from build123d import *

# Parameters (mm, degrees)
BOSS_EXTRUDE1_DEPTH = 1.6
SKETCH2_R           = 2.55
SKETCH2_R_2         = 3.6
CUT_EXTRUDE1_DEPTH  = 1.6
SKETCH3_R           = 1.55
CUT_EXTRUDE2_DEPTH  = 1.6


with BuildPart() as part:
    # Sketch1 → Boss-Extrude1 (new body)
    with BuildSketch(Plane(origin=(0, 0, 0), x_dir=(1, 0, 0), z_dir=(0, 1, 0))):
        with BuildLine():
            Line((-26.8, 32.5), (26.8, 32.5))
            ThreePointArc((26.8, 32.5), (34.366042559, 29.366042559), (37.5, 21.8))
            Line((37.5, 21.8), (37.5, -21.8))
            ThreePointArc((37.5, -21.8), (34.366042559, -29.366042559), (26.8, -32.5))
            Line((26.8, -32.5), (-26.8, -32.5))
            ThreePointArc((-26.8, -32.5), (-34.366042559, -29.366042559), (-37.5, -21.8))
            Line((-37.5, -21.8), (-37.5, 21.8))
            ThreePointArc((-37.5, 21.8), (-34.366042559, 29.366042559), (-26.8, 32.5))
        make_face()
    extrude(amount=BOSS_EXTRUDE1_DEPTH)

    # Sketch2 → Cut-Extrude1 (cut)
    with BuildSketch(Plane(origin=(0, 1.6, 0), x_dir=(1, 0, 0), z_dir=(0, 1, 0))):
        with Locations(Location((25.95, 25, 0), (0, 0, 270))):
            Circle(SKETCH2_R)
        with Locations(Location((25.95, -25, 0), (0, 0, 270))):
            Circle(SKETCH2_R)
        with Locations(Location((-25.95, -25, 0), (0, 0, 270))):
            Circle(SKETCH2_R_2)
        with Locations(Location((-25.95, 25, 0), (0, 0, 270))):
            Circle(SKETCH2_R_2)
    extrude(amount=-CUT_EXTRUDE1_DEPTH, mode=Mode.SUBTRACT)

    # Sketch3 → Cut-Extrude2 (cut)
    with BuildSketch(Plane(origin=(0, 1.6, 0), x_dir=(1, 0, 0), z_dir=(0, 1, 0))):
        with Locations(Location((-30, 0, 0), (0, 0, 270))):
            Circle(SKETCH3_R)
        with Locations(Location((30, 0, 0), (0, 0, 270))):
            Circle(SKETCH3_R)
    extrude(amount=-CUT_EXTRUDE2_DEPTH, mode=Mode.SUBTRACT)


solid = part.part
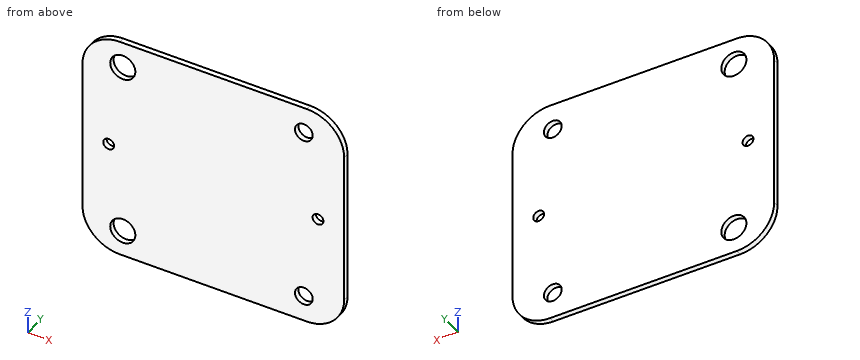
Build history of the part. All positions in model axes, mm. Coordinates: 2 decimals unless noted, no trailing zeros. Order: outer loops, then holes, each group sorted by start corner. A loop starts at its lowest first (then second) coordinate and runs counter-clockwise, first axis right, second up. Notation, with made-up numbers: (-10, 45) - (28, 45) arc R13 cw to (28, 66) - close; hole circle Ø10 at (59.25, 40). An arc over 180 degrees is marked (long way). Write each question's results on one line, items separated by ' | '. Start each with the question number.
Item 1: Flat gauge pin, fed straight in: pin 1 (4 mm diameter, centred on x = 25.95, z = 25, fed in from +Y). Where does the tip first touch, or does it go through?
Item 2: Band-saw the part on A-A on x = 25.95. Write the cut outline in (y, z), and give its area (3 significant figures).
Item 3: Wall check: probe 1 along X at (y, z) = (0.8, 0); probe 2 along X at (y, z) = (0.75, 25); probe 3 along Z at (x, y) = (-23.5, 1.35). Give the ranges that are in metal, low to high. Write a range as [from, to].
Item 4: Band-saw the part on B-B on z = -25. Write the cut outline in (x, y), and give its area (3 significant figures).
Item 5: Band-saw the part on C-C on y = 0.35. Write the cut outline in (x, z), and give its area (3 significant figures).
Numbers:
1) pin 1: through
2) outline: (0, -32.5) - (1.6, -32.5) - (1.6, -27.55) - (0, -27.55) - close; (0, -22.45) - (1.6, -22.45) - (1.6, 22.45) - (0, 22.45) - close; (0, 27.55) - (1.6, 27.55) - (1.6, 32.5) - (0, 32.5) - close | area: 87.7 mm^2
3) probe 1: [-37.5, -31.55], [-28.45, 28.45], [31.55, 37.5] | probe 2: [-37.01, -29.55], [-22.35, 23.4], [28.5, 37.01] | probe 3: [-32.5, -27.64], [-22.36, 22.36], [27.64, 32.5]
4) outline: (-37.01, 0) - (-29.55, 0) - (-29.55, 1.6) - (-37.01, 1.6) - close; (-22.35, 0) - (23.4, 0) - (23.4, 1.6) - (-22.35, 1.6) - close; (28.5, 0) - (37.01, 0) - (37.01, 1.6) - (28.5, 1.6) - close | area: 98.8 mm^2
5) outline: (-37.5, -21.8) arc R10.7 ccw to (-26.8, -32.5) - (26.8, -32.5) arc R10.7 ccw to (37.5, -21.8) - (37.5, 21.8) arc R10.7 ccw to (26.8, 32.5) - (-26.8, 32.5) arc R10.7 ccw to (-37.5, 21.8) - close; hole circle Ø3.1 at (-30, 0); hole circle Ø7.2 at (-25.95, -25); hole circle Ø7.2 at (-25.95, 25); hole circle Ø5.1 at (25.95, -25); hole circle Ø5.1 at (25.95, 25); hole circle Ø3.1 at (30, 0) | area: 4,640 mm^2
